Here's how the part is built. I have some questions about the finished solid (model axes, mm). A direction names the side the tool comes from. Round coordinates to 2 decimals unless told otherwise and drop trailing zeros. Write each loop counter-clockwise with the first axis right and the second up, starting at its lowest first coordinate (ties: lowest second). Pieces come first, ordered by that corner, then holes. Notation, with made-up numbers: (3, 9.5) -> (50, 9.5) arc R27 cw to (50, 29.5) -> close; hole circle Ø3 at (-16.75, -36). An arc over 180 degrees is marked (long way). Answer in a Markdown table with one row per item.
from build123d import *

# Parameters (mm, degrees)
ESBO_O1_W                = 50
ESBO_O1_H                = 20
ESBO_O1_R                = 3
RESSALTO_EXTRUS_O1_DEPTH = 15
ESBO_O2_R                = 2
CORTE_EXTRUS_O1_DEPTH    = 56.402686144
ESBO_O3_R                = 2
CORTE_EXTRUS_O2_DEPTH    = 4


with BuildPart() as part:
    # Esboço1 → Ressalto-extrusão1 (new body)
    with BuildSketch(Plane(origin=(0, 0, 0), x_dir=(1, 0, 0), z_dir=(0, 1, 0))):
        with Locations((24.441456613, 31)):
            Rectangle(ESBO_O1_W, ESBO_O1_H)
        with Locations(Location((10.241456613, 35.210777548, 0), (0, 0, 270))):
            Circle(ESBO_O1_R, mode=Mode.SUBTRACT)
        with Locations(Location((38.641456613, 35.210777548, 0), (0, 0, 270))):
            Circle(ESBO_O1_R, mode=Mode.SUBTRACT)
    extrude(amount=RESSALTO_EXTRUS_O1_DEPTH)

    # Esboço2 → Corte-extrusão1 (cut, through all)
    with BuildSketch(Plane(origin=(0, 0, -41), x_dir=(-1, 0, 0), z_dir=(0, 0, -1))):
        with Locations((-3.441456613, 7.5)):
            Circle(ESBO_O2_R)
        with Locations((-45.441456613, 7.5)):
            Circle(ESBO_O2_R)
    extrude(amount=-CORTE_EXTRUS_O1_DEPTH, mode=Mode.SUBTRACT)

    # Esboço3 → Corte-extrusão2 (cut)
    with BuildSketch(Plane(origin=(0, 0, -41), x_dir=(-1, 0, 0), z_dir=(0, 0, -1))):
        with Locations((-10.241456613, 7.5)):
            Circle(ESBO_O3_R)
        with Locations((-38.641456613, 7.5)):
            Circle(ESBO_O3_R)
    extrude(amount=-CORTE_EXTRUS_O2_DEPTH, mode=Mode.SUBTRACT)


solid = part.part
1) I want a section at B-B, the plane z = -26.25. List the corners of the cut face in (x, y) for me.
Response:
| item | result |
|---|---|
| outline | (-0.56, 0) -> (49.44, 0) -> (49.44, 15) -> (-0.56, 15) -> close; hole circle Ø4 at (3.44, 7.5); hole circle Ø4 at (45.44, 7.5) |
2) For pin 1 (5 mm diameter, centred on x = 38.64, z = -35.21, fed in from +Y); pin 2 (1 mm diameter, centred on x = 17.5, z = -37, fed in from -Y); pin 3 (3 mm diameter, centred on x = 38.64, y = 7.5, fed in from -Z), each with a flat end and sliding along its axis, tell me the tip position at first contact or that it passes through.
Response:
| item | result |
|---|---|
| pin 1 | passes through |
| pin 2 | stops at y = 0 |
| pin 3 | stops at z = -32.61 |
3) I need wall thicknesses on line 1 (Z direction, x = 10.5, y = 2.5); line 2 (X direction, y = 12.5, z = -33.25); line 3 (X direction, y = 11.5, z = -33). Which ranges of each line are inside material? Lowest first, please. Write a range as [from, to].
Response:
| item | result |
|---|---|
| line 1 | z = [-41, -38.2], [-32.22, -21] |
| line 2 | x = [-0.56, 7.97], [12.51, 36.37], [40.91, 49.44] |
| line 3 | x = [-0.56, 8.21], [12.27, 36.61], [40.67, 49.44] |
4) We'd pull the mould along Z, two halves only. Please class faces 3 (the face through (24, 7, -41)), 4 (the face through (24, 7, -21)), 5 (the face through (11.14, 7.4, -32.35)), 6 (the face through (2.37, 9.19, -31.14)): +Z half, -Z half, draft (parallel to the pull), parting line (faces both ways), or undercut.
Response:
| item | result |
|---|---|
| face 3 | -Z half |
| face 4 | +Z half |
| face 5 | undercut |
| face 6 | draft |
5) I want a section at A-A, the plane y = 7.5. List the corners of the cut face in (x, z) for me.
Response:
| item | result |
|---|---|
| outline | (-0.56, -41) -> (1.44, -41) -> (1.44, -21) -> (-0.56, -21) -> close; (5.44, -41) -> (8.24, -41) -> (8.24, -37.45) arc R3 cw (long way) to (12.24, -37.45) -> (12.24, -41) -> (36.64, -41) -> (36.64, -37.45) arc R3 cw (long way) to (40.64, -37.45) -> (40.64, -41) -> (43.44, -41) -> (43.44, -21) -> (5.44, -21) -> close; (47.44, -41) -> (49.44, -41) -> (49.44, -21) -> (47.44, -21) -> close |
6) Which directions (+Z, -Z, +X, -X, +Y, -Y) give clear straight access to the entire face, cutting with the end or side of a thin tool? Please do faces 1 (the face through (-0.559, 7, -31)), 2 (the face through (37.57, 9.19, -39.25)).
Response:
| item | result |
|---|---|
| face 1 | +Z, -Z, -X, +Y, -Y |
| face 2 | -Z |
7) I want a section at C-C, the plane y = 2.5. List the corners of the cut face in (x, z) for me.
Response:
| item | result |
|---|---|
| outline | (-0.56, -41) -> (49.44, -41) -> (49.44, -21) -> (-0.56, -21) -> close; hole circle Ø6 at (10.24, -35.21); hole circle Ø6 at (38.64, -35.21) |
